Verification items for the finished model (mm, model axes). A direction names the side the tool comes from. Round coordinates to 2 decimals unless told otherwise and drop trailing zeros. Write each loop counter-clockwise with the first axis right and the second up, starting at its lowest first coordinate (ties: lowest second). Pieces come first, ordered by that corner, then holes. Notation, with made-up numbers: M -30.75,29.5 L -25.75,29.5 A17 ccw -25.75,59.5 Z; hole C 42,83 d8. An arc over 180 degrees is marked long. One line per item, written item: value. Start each with the question number.
Item 1: Thickness scan on probe 1 along X at (y, z) = (11, 42) (3 decimals); probe 2 along Y at (x, z) = (20.75, 19.5) (3 decimals). Record the ranges inside material, lowest first. Write a range as from..to.
Item 2: Section check D-D, the plane z = 39. Record the cut outline in (x, y) (3 decimals).
Item 3: Section check B-B, the plane z = 19.5. Record the cut outline in (x, y) (3 decimals), then the cut area to 3 significant figures.
Item 4: Section check A-A, the plane x = 24. Record the cut outline in (y, z) (3 decimals).
Item 5: Draft check along Z on faces 1 (the face through (9, 26, 0)), 2 (the face through (25.2, 27, 17.7)), 3 (the face through (3.175, 13, 31)). Enter one of: +Z half, -Z half, draft (parallel to the pull), parting line (faces both ways), or undercut.
Item 6: Gauge pin test, flat ends, axial feed: pin 1 (8 mm diameter, centred on y = 16, z = 12.5, fed in from +X) (3 decimals); pin 2 (12 mm diameter, centred on x = 13.5, z = 47.5, fed in from -Y). Record the tip position at first contact, or that the pin passes through.
Item 7: Section check C-C, the plane x = 18.75. Record the cut outline in (y, z) (3 decimals), then the cut area to 3 significant figures.
Item 8: Tool access check on faces 4 (the face through (28.575, 27, 31)), 5 (the face through (16, 25.4, 31)). Record the directions out of +Z, -Z, +X, -X, +Y, -Y that give a thin tool (end or side, any length) a straight path to the whole face; none if there is none.
from build123d import *

# Parameters (mm, degrees)
BOSS_EXTRUDE1_DEPTH = 63.5
CUT_EXTRUDE1_REACH  = 30.575
SKETCH2_R           = 2.0193


with BuildPart() as part:
    # Sketch1 → Boss-Extrude1 (new body)
    with BuildSketch(Plane.XY):
        Polygon((0, 0), (0, 28.575), (28.575, 28.575), (28.575, 25.4), (3.175, 25.4), (3.175, 0), align=None)
    extrude(amount=BOSS_EXTRUDE1_DEPTH)

    # Sketch2 → Cut-Extrude1 (cut, up to next)
    with BuildSketch(Plane(origin=(0, 28.575, 0), x_dir=(1, 0, 0), z_dir=(0, 1, 0)), mode=Mode.PRIVATE) as cut_extrude1_sk1:
        with Locations((23.275, -43.710246093)):
            Circle(SKETCH2_R)
    cut_extrude1_tool1 = extrude(cut_extrude1_sk1.sketch, amount=-CUT_EXTRUDE1_REACH, mode=Mode.PRIVATE) & part.part
    add(cut_extrude1_tool1.solids().sort_by_distance((23.275, 28.575, 43.710246))[0], mode=Mode.SUBTRACT)
    # Sketch2 → Cut-Extrude1 (cut, up to next)
    with BuildSketch(Plane(origin=(0, 28.575, 0), x_dir=(1, 0, 0), z_dir=(0, 1, 0)), mode=Mode.PRIVATE) as cut_extrude1_sk2:
        with Locations((23.275, -18.310246093)):
            Circle(SKETCH2_R)
    cut_extrude1_tool2 = extrude(cut_extrude1_sk2.sketch, amount=-CUT_EXTRUDE1_REACH, mode=Mode.PRIVATE) & part.part
    add(cut_extrude1_tool2.solids().sort_by_distance((23.275, 28.575, 18.310246))[0], mode=Mode.SUBTRACT)


solid = part.part
Response values:
1. probe 1: x = 0..3.175
1. probe 2: y = 25.4..28.575
2. outline: M 0,0 L 3.175,0 L 3.175,25.4 L 28.575,25.4 L 28.575,28.575 L 0,28.575 Z
3. outline: M 0,0 L 3.175,0 L 3.175,25.4 L 21.643,25.4 L 21.643,28.575 L 0,28.575 Z; M 24.907,25.4 L 28.575,25.4 L 28.575,28.575 L 24.907,28.575 Z
3. area: 161 mm2
4. outline: M 25.4,0 L 28.575,0 L 28.575,16.426 L 25.4,16.426 Z; M 25.4,20.195 L 28.575,20.195 L 28.575,41.826 L 25.4,41.826 Z; M 25.4,45.595 L 28.575,45.595 L 28.575,63.5 L 25.4,63.5 Z
5. face 1: -Z half
5. face 2: undercut
5. face 3: draft
6. pin 1: stops at x = 3.175
6. pin 2: stops at y = 25.4
7. outline: M 25.4,0 L 28.575,0 L 28.575,63.5 L 25.4,63.5 Z
7. area: 202 mm2
8. face 4: +Z, -Z, +X, +Y, -Y
8. face 5: +Z, -Z, +X, -Y
